```python
from build123d import *

# Parameters (mm, degrees)
BOSS_EXTRUDE1_DEPTH = 10
CUT_EXTRUDE16_DEPTH = 10


with BuildPart() as part:
    # Sketch1 → Boss-Extrude1 (new body)
    with BuildSketch(Plane.XY):
        with BuildLine():
            Line((-50, 60), (50, 60))
            ThreePointArc((50, 60), (57.071067812, 57.071067812), (60, 50))
            Line((60, 50), (60, -50))
            ThreePointArc((60, -50), (57.071067812, -57.071067812), (50, -60))
            Line((50, -60), (-50, -60))
            ThreePointArc((-50, -60), (-57.071067812, -57.071067812), (-60, -50))
            Line((-60, -50), (-60, 50))
            ThreePointArc((-60, 50), (-57.071067812, 57.071067812), (-50, 60))
        make_face()
    extrude(amount=BOSS_EXTRUDE1_DEPTH)

    # Sketch2 → Cut-Extrude16 (cut)
    with BuildSketch(Plane.XY.offset(10)):
        with BuildLine():
            Line((41.217948718, 31.01963141), (28.71494391, 19.068509615))
            add(Edge.make_bspline(
                [(28.71494391, 19.068509615), (27.654337183, 20.165178749), (25.582639967, 22.307317142), (22.244356118, 25.143319595), (18.772662463, 27.506743914), (15.235093873, 29.497204828), (11.568019744, 31.00313037), (7.813841439, 32.100523678), (3.948587424, 32.7695629), (1.332732176, 32.846112827), (0.017027244, 32.884615385)],
                knots=[0, 0, 0, 0, 1.115251505, 2.178435587, 3.19620269, 4.182487026, 5.141301733, 6.088180966, 7.038406374, 8, 8, 8, 8], degree=3))
            add(Edge.make_bspline(
                [(0.017027244, 32.884615385), (-1.081746264, 32.854197018), (-3.250054721, 32.794169724), (-6.433699741, 32.354110448), (-9.479020737, 31.605770498), (-12.396442325, 30.574419427), (-15.177379867, 29.239905879), (-17.827663943, 27.603262735), (-20.340760389, 25.679271209), (-22.683472657, 23.477886123), (-24.826503507, 21.072707488), (-26.720007718, 18.506387623), (-28.30612123, 15.784805822), (-29.60781879, 12.935524265), (-30.621790871, 9.945355068), (-31.345894329, 6.816311329), (-31.764696418, 3.544666601), (-31.827205437, 1.320626893), (-31.858974359, 0.190304487)],
                knots=[0, 0, 0, 0, 1.035432265, 2.043311493, 3.022114605, 3.98653278, 4.95457646, 5.923598177, 6.917315552, 7.932509744, 8.948865224, 9.949768934, 10.933144597, 11.912367597, 12.897413939, 13.903909035, 14.934704909, 16, 16, 16, 16], degree=3))
            add(Edge.make_bspline(
                [(-31.858974359, 0.190304487), (-31.849818918, -0.603034863), (-31.831773356, -2.166723023), (-31.634232763, -4.479851798), (-31.316145828, -6.72413356), (-30.855795226, -8.896168818), (-30.280122272, -10.997839879), (-29.604726818, -13.047277753), (-28.757453155, -15.016163821), (-27.816966606, -16.927365418), (-26.723191587, -18.728733016), (-25.543900342, -20.44648652), (-24.265151526, -22.072205676), (-22.878662607, -23.599244492), (-21.364920479, -25.003738772), (-19.763049776, -26.32792333), (-18.046029154, -27.538649342), (-16.249525485, -28.66630131), (-14.358019245, -29.645902168), (-12.422831386, -30.533231294), (-10.414620559, -31.25387447), (-8.357837936, -31.834778614), (-6.259833735, -32.328750831), (-4.100087524, -32.632904706), (-1.8973216, -32.863236875), (-0.408621569, -32.87745854), (0.340544872, -32.884615385)],
                knots=[0, 0, 0, 0, 1.103660481, 2.175337485, 3.227646561, 4.255952547, 5.262355991, 6.258840057, 7.255597736, 8.242457506, 9.22035537, 10.185017736, 11.140346927, 12.096287581, 13.051739095, 14.01125915, 14.986044842, 15.97314143, 16.960198552, 17.947847494, 18.933482797, 19.925264591, 20.920966487, 21.929612487, 22.958107872, 24, 24, 24, 24], degree=3))
            add(Edge.make_bspline(
                [(0.340544872, -32.884615385), (1.611259903, -32.847859563), (4.107884503, -32.77564393), (7.772040087, -32.210927911), (11.263615319, -31.282002017), (14.053367221, -30.184994512), (16.239064148, -29.101685359), (17.903002908, -28.09967774), (19.623645272, -26.978822204), (21.372412843, -25.696816449), (23.168975786, -24.269045058), (24.981620624, -22.664237173), (26.856751385, -20.935236817), (28.08513096, -19.701215296), (28.71494391, -19.068509615)],
                knots=[0, 0, 0, 0, 1.404581149, 2.759636711, 4.088442092, 5.392261763, 6.066678138, 6.783632037, 7.538459478, 8.336747902, 9.180226004, 10.074962426, 11.012997595, 12, 12, 12, 12], degree=3))
            Line((28.71494391, -19.068509615), (40.837339744, -31.799879808))
            add(Edge.make_bspline(
                [(40.837339744, -31.799879808), (39.985200566, -32.622593431), (38.322007128, -34.228354481), (35.813125998, -36.508385331), (33.307402394, -38.557246511), (30.865369379, -40.449302703), (28.447023904, -42.129433712), (26.052622431, -43.599317508), (23.709270632, -44.896129576), (21.368308056, -45.997999818), (19.015168024, -46.933602094), (16.594063463, -47.739094243), (14.097592829, -48.420511624), (11.510508817, -48.970325958), (8.856942171, -49.411202829), (6.112059034, -49.708792168), (3.293263318, -49.908851579), (1.381230514, -49.926828575), (0.416666667, -49.935897436)],
                knots=[0, 0, 0, 0, 1.244526981, 2.429050516, 3.560637417, 4.644440555, 5.67424972, 6.652764056, 7.595344123, 8.486817594, 9.369275933, 10.254498637, 11.166417451, 12.086725134, 13.032340136, 13.991389299, 14.986715468, 16, 16, 16, 16], degree=3))
            add(Edge.make_bspline(
                [(0.416666667, -49.935897436), (-1.35511764, -49.89073112), (-4.822007032, -49.802353196), (-9.902643041, -49.147532612), (-14.729110869, -48.049737439), (-19.313152407, -46.497152269), (-23.653310037, -44.513797477), (-27.748473415, -42.082297632), (-31.592042048, -39.209112847), (-35.152967466, -35.927919636), (-38.373993978, -32.304117189), (-41.221008401, -28.413147516), (-43.576058839, -24.235887927), (-45.531507964, -19.834049889), (-47.060643461, -15.187546107), (-48.136895621, -10.291350477), (-48.800612473, -5.150190581), (-48.87322404, -1.638659859), (-48.91025641, 0.15224359)],
                knots=[0, 0, 0, 0, 1.078019885, 2.10938526, 3.111377082, 4.085535484, 5.04941344, 6.010039228, 6.978205633, 7.964457913, 8.951525778, 9.924444315, 10.892603023, 11.863865945, 12.85144698, 13.863884204, 14.910567087, 16, 16, 16, 16], degree=3))
            add(Edge.make_bspline(
                [(-48.91025641, 0.15224359), (-48.894608325, 1.320255539), (-48.863597646, 3.634969751), (-48.537672531, 7.044731317), (-48.08331397, 10.368638931), (-47.362515429, 13.572179417), (-46.493663878, 16.698510375), (-45.41313282, 19.713652236), (-44.122648013, 22.626270824), (-42.663804821, 25.441242036), (-41.013430113, 28.140124795), (-39.169780387, 30.699731445), (-37.180318376, 33.139821677), (-34.99724055, 35.428023165), (-32.652269888, 37.584426764), (-30.134819118, 39.597346508), (-27.460029448, 41.495649937), (-24.620661217, 43.230384415), (-21.671875784, 44.799543954), (-18.650865094, 46.183609685), (-15.565051419, 47.340369909), (-12.42748186, 48.299859845), (-9.224900224, 49.016051238), (-5.980165725, 49.558185018), (-2.665669568, 49.861241267), (-0.440272542, 49.910853509), (0.683092949, 49.935897436)],
                knots=[0, 0, 0, 0, 1.071919942, 2.124283339, 3.142214191, 4.149696895, 5.136002878, 6.119640489, 7.086990633, 8.058538607, 9.028339693, 9.988281803, 10.952401235, 11.916291999, 12.888973767, 13.874849856, 14.873389453, 15.898127285, 16.927174885, 17.938320013, 18.946391617, 19.950418109, 20.947802303, 21.956882652, 22.968648068, 24, 24, 24, 24], degree=3))
            add(Edge.make_bspline(
                [(0.683092949, 49.935897436), (1.641438895, 49.921541632), (3.548166658, 49.892979285), (6.387604259, 49.654881043), (9.204333367, 49.280950163), (11.988269228, 48.716768097), (14.759325397, 48.047012689), (17.481087091, 47.170060366), (20.196491572, 46.192531741), (22.862951754, 45.024095868), (25.484189625, 43.74864257), (27.998798557, 42.301594484), (30.448998604, 40.772001333), (32.780494803, 39.069335094), (35.036961098, 37.255354635), (37.206598229, 35.321596721), (39.270366363, 33.235819929), (40.565472654, 31.7620955), (41.217948718, 31.01963141)],
                knots=[0, 0, 0, 0, 0.996412454, 1.982464992, 2.961075852, 3.949442424, 4.934965278, 5.923860011, 6.921385422, 7.934793307, 8.949617135, 9.951082467, 10.950285876, 11.951772932, 12.951063433, 13.960125323, 14.972308753, 16, 16, 16, 16], degree=3))
        make_face()
    extrude(amount=-CUT_EXTRUDE16_DEPTH, mode=Mode.SUBTRACT)


solid = part.part
```
Part model, mm, in its own coordinate system. A direction names the side the tool comes from. Round coordinates to 2 decimals unless told otherwise and drop trailing zeros.
1. 3-axis set-ups, long thin cutter, end or side, ignore diameter. For faces 1 (the face through (35.054, 25.128, 5.07)), 2 (the face through (60, 1, 5)): which of +Z, -Z, +X, -X, +Y, -Y reach the whole face in a straight line?
Solutions:
face 1: +Z, -Z
face 2: +Z, -Z, +X, +Y, -Y
2. Drill centre lines: line 1 along X through (y, z) = (-25, 6); line 2 along Y through (x, z) = (9, 4); line 3 along Y through (x, z) = (35.5, 5.25). Where is each one in solid material? Low to high.
Solutions:
line 1: x = -60 to -43.1, -21.34 to 22.24, 34.36 to 60
line 2: y = -60 to -49.37, -31.86 to 31.73, 49.28 to 60
line 3: y = -60 to -36.74, -26.19 to 25.55, 36.83 to 60
3. Slice it at A-A (x = 11.5). Count the separate pieces of the cut face and the enclosed holes in it, and give its area (3 significant figures).
Solutions:
separate pieces: 3
enclosed holes: 0
area: 843 mm2
